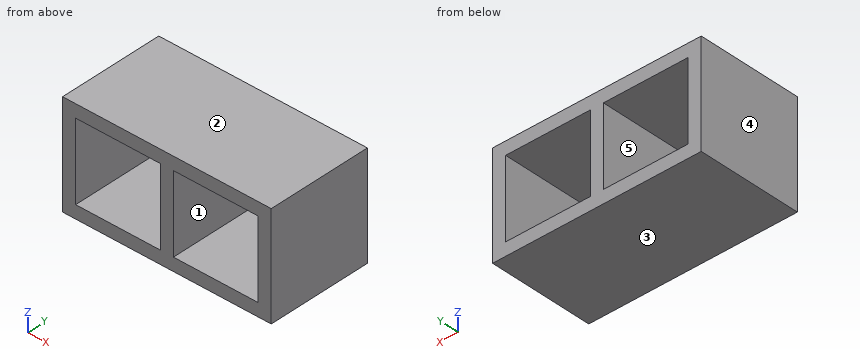
from build123d import *

# Parameters (mm, degrees)
F0_W     = 406.4
F0_H     = 203.2
F1_DEPTH = 203.2
F2_W     = 165.1
F2_H     = 152.4
F3_DEPTH = 203.201
F4_DEPTH = 203.201


with BuildPart() as f1:
    # F0 (on Top) → F1 (new body)
    with BuildSketch(Plane.XY):
        with Locations((203.2, 101.6)):
            Rectangle(F0_W, F0_H)
    extrude(amount=F1_DEPTH)

    # F2 (on face) → F3 (cut, through all)
    with BuildSketch(Plane.XZ):
        with Locations((107.95, 101.6)):
            Rectangle(F2_W, F2_H)
        with Locations((298.45, 101.6)):
            Rectangle(F2_W, F2_H)
    extrude(amount=-F3_DEPTH, mode=Mode.SUBTRACT)

    # F2 (on face) → F4 (cut, through all)
    with BuildSketch(Plane.XZ):
        with Locations((107.95, 101.6)):
            Rectangle(F2_W, F2_H)
        with Locations((298.45, 101.6)):
            Rectangle(F2_W, F2_H)
    extrude(amount=-F4_DEPTH, mode=Mode.SUBTRACT)


solid = f1.part
Input: part model. Units: mm. Frame: model coordinates. Face numbers are marked on the shaded views. A direction names the side the tool comes from. Round coordinates to 2 decimals unless told otherwise and drop trailing zeros. Order: outer loops, then holes, each group sorted by start corner. A loop starts at its lowest first (then second) coordinate and runs counter-clockwise, first axis right, second up. Notation, with made-up numbers: (-12.5, 67) - (36.5, 67) arc R31 ccw to (36.5, 93) - close; hole circle Ø11 at (42.5, 74). An arc over 180 degrees is marked (long way). Answer as a JSON object with one key per item and string values. Group by question number.
(1) Cut plane B-B (x = 157). Return loops of the section in (y, z), then the cut area to 3 significant figures.
(2) Cut plane C-C (y = 17.5). Return loops of the section in (x, z), then the cut area to 3 significant figures.
(3) Pin query (flat end, axial travel): P1, Ø10, axis at x = 102, y = 37.5, coming from the -Z side. Return the tip coordinate at first contact, or that it passes through.
(4) Draft query along Z for the marked faces 3, 4 and 5. Return one class per face: released by +Z, released by -Z, zero draft, split by the parting line, or undercut.
(5) Reachability of the marked faces 1 and 2 from +Z, -Z, +X, -X, +Y, -Y: full face, straight path, thin tool, end or side. Return the list, or none.
(6) Cut plane A-A (z = 164.5). Return loops of the section in (x, y).
(7) Material intervals for probe 1 along X at (y, z) = (170, 63); probe 2 along Z at (x, y) = (352, 193), sorted ascending. Write a range as from..to.
Here are the results:
{
 "1": {"outline": "(0, 0) - (203.2, 0) - (203.2, 25.4) - (0, 25.4) - close; (0, 177.8) - (203.2, 177.8) - (203.2, 203.2) - (0, 203.2) - close", "area": "10,300 mm^2"},
 "2": {"outline": "(0, 0) - (406.4, 0) - (406.4, 203.2) - (0, 203.2) - close; hole (25.4, 25.4) - (190.5, 25.4) - (190.5, 177.8) - (25.4, 177.8) - close; hole (215.9, 25.4) - (381, 25.4) - (381, 177.8) - (215.9, 177.8) - close", "area": "32,300 mm^2"},
 "3": {"P1": "stops at z = 0"},
 "4": {"face 3": "released by -Z", "face 4": "zero draft", "face 5": "undercut"},
 "5": {"face 1": "+Y, -Y", "face 2": "+Z, +X, -X, +Y, -Y"},
 "6": {"outline": "(0, 0) - (25.4, 0) - (25.4, 203.2) - (0, 203.2) - close; (190.5, 0) - (215.9, 0) - (215.9, 203.2) - (190.5, 203.2) - close; (381, 0) - (406.4, 0) - (406.4, 203.2) - (381, 203.2) - close"},
 "7": {"probe 1": "x = 0..25.4, 190.5..215.9, 381..406.4", "probe 2": "z = 0..25.4, 177.8..203.2"}
}
